```python
from build123d import *

# Parameters (mm, degrees)
F0_R     = 30
F1_DEPTH = 6.35
F3_D     = 10
F5_D     = 6.6
F6_D     = 2.7051
F7_D     = 2.7051
F9_D     = 6.35
F10_D    = 2.7051


with BuildPart() as f1:
    # F0 (on Top) → F1 (new body)
    with BuildSketch(Plane.XY):
        Polygon((-180, 60), (-120, 0), (120, 0), (180, 60), (180, 220), (120, 280), (-120, 280), (-180, 220), align=None)
        with Locations((0, 140)):
            Circle(F0_R, mode=Mode.SUBTRACT)
    extrude(amount=F1_DEPTH)

    # F3 (through all)
    with Locations(Plane.XY.offset(6.35)):
        with Locations((-125, 140), (125, 140)):
            Hole(F3_D / 2)

    # F5 (through all)
    with Locations(Plane.XY.offset(6.35)):
        with Locations((-121.2489651369, 251.2489651369), (-151.2489651369, 221.2489651369), (-151.2489651369, 58.7510348631), (-121.2489651369, 28.7510348631), (121.2489651369, 28.7510348631), (151.2489651369, 58.7510348631), (151.2489651369, 221.2489651369), (121.2489651369, 251.2489651369)):
            Hole(F5_D / 2)

    # F6 (through all)
    with Locations(Plane.XY.offset(6.35)):
        with Locations((-150, 235.8578643763), (-135.8578643763, 250)):
            Hole(F6_D / 2)

    # F7 (through all)
    with Locations(Plane.XY.offset(6.35)):
        with Locations((-150, 44.1421356237), (-135.8578643763, 30), (135.8578643763, 250), (150, 235.8578643763), (135.8578643763, 30), (150, 44.1421356237)):
            Hole(F7_D / 2)

    # F9 (through all)
    with Locations(Plane.XY.offset(6.35)):
        with Locations((0, 208.14583), (59.016019942, 174.072915), (-59.016019942, 174.072915), (-59.016019942, 105.927085), (0, 71.85417), (59.016019942, 105.927085)):
            Hole(F9_D / 2)

    # F10 (through all)
    with Locations(Plane.XY.offset(6.35)):
        with Locations((147.7549359697, 247.7549359697), (147.7549359697, 32.2450640303), (-147.7549359697, 32.2450640303), (-147.7549359697, 247.7549359697)):
            Hole(F10_D / 2)


solid = f1.part
```
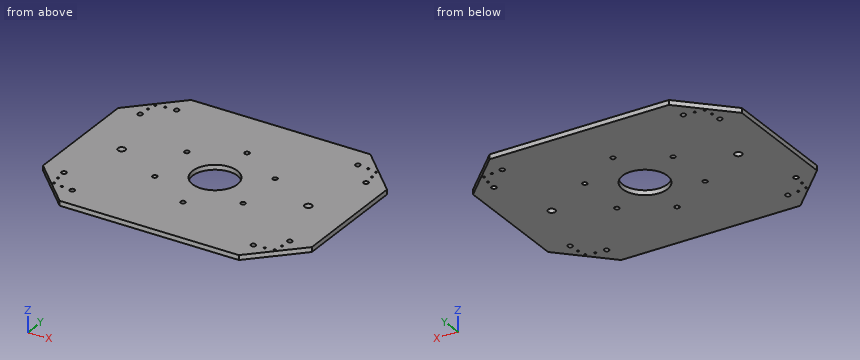
For this review, take the finished solid that the model builds, in its own axes (mm). Round coordinates to 2 decimals unless told otherwise and drop trailing zeros. Write each loop counter-clockwise with the first axis right and the second up, starting at its lowest first coordinate (ties: lowest second). Pieces come first, ordered by that corner, then holes. Notation, with made-up numbers: M 31.5,-8 L 65.5,-8 A22 ccw 65.5,8 Z; hole C -33,36 d6. An arc over 180 degrees is marked long. One line per item, written item: value. Start each with the question number.
(1) We need section A-A (y = 140). Give the boundary of the cut face in (x, z).
(2) We need section B-B (z = 4). Count the separate pieces of the cut face and the enclosed holes in it, and give its area (3 significant figures).
(3) Wall thickness on line 1 (Y direction, x = -61, z = 3.75); line 2 (X direction, y = 175.5, z = 4); line 3 (X direction, y = 58.5, z = 0.5): over which ranges is each line inside the solid? List them lowest first.
(4) Insertion check: pin 1 (1.6 mm diameter, centred on x = -135.86, y = 250, fed in from -Z). The pin has a flat end and moves straight along its axis. Give the tip position at first contact, or say it passes through.
Result:
1. outline: M -180,0 L -130,0 L -130,6.35 L -180,6.35 Z; M -120,0 L -30,0 L -30,6.35 L -120,6.35 Z; M 30,0 L 120,0 L 120,6.35 L 30,6.35 Z; M 130,0 L 180,0 L 180,6.35 L 130,6.35 Z
2. separate pieces: 1
2. enclosed holes: 29
2. area: 90,100 mm²
3. line 1: 0 to 103.45, 108.41 to 171.59, 176.55 to 280
3. line 2: -180 to -61.85, -56.18 to 56.18, 61.85 to 180
3. line 3: -178.5 to -154.54, -147.96 to 147.96, 154.54 to 178.5
4. pin 1: through
